Input: dimensioned drawing with shaded views. Units: mm. Origin: part minimum x, y, z. A direction names the side the tool comes from. Round coordinates to 2 decimals unless told otherwise and drop trailing zeros. Loops run counter-clockwise (first coordinate to the right, second up) from the corner with the lowest first, then second, coordinate; pieces in that order, holes last. Notation, with made-up numbers: M 84,16.25 L 138,16.25 A22 cw 138,43.25 Z; hole C 36.5,68.5 d10. An arc over 180 degrees is marked long. One line per item, written item: value.
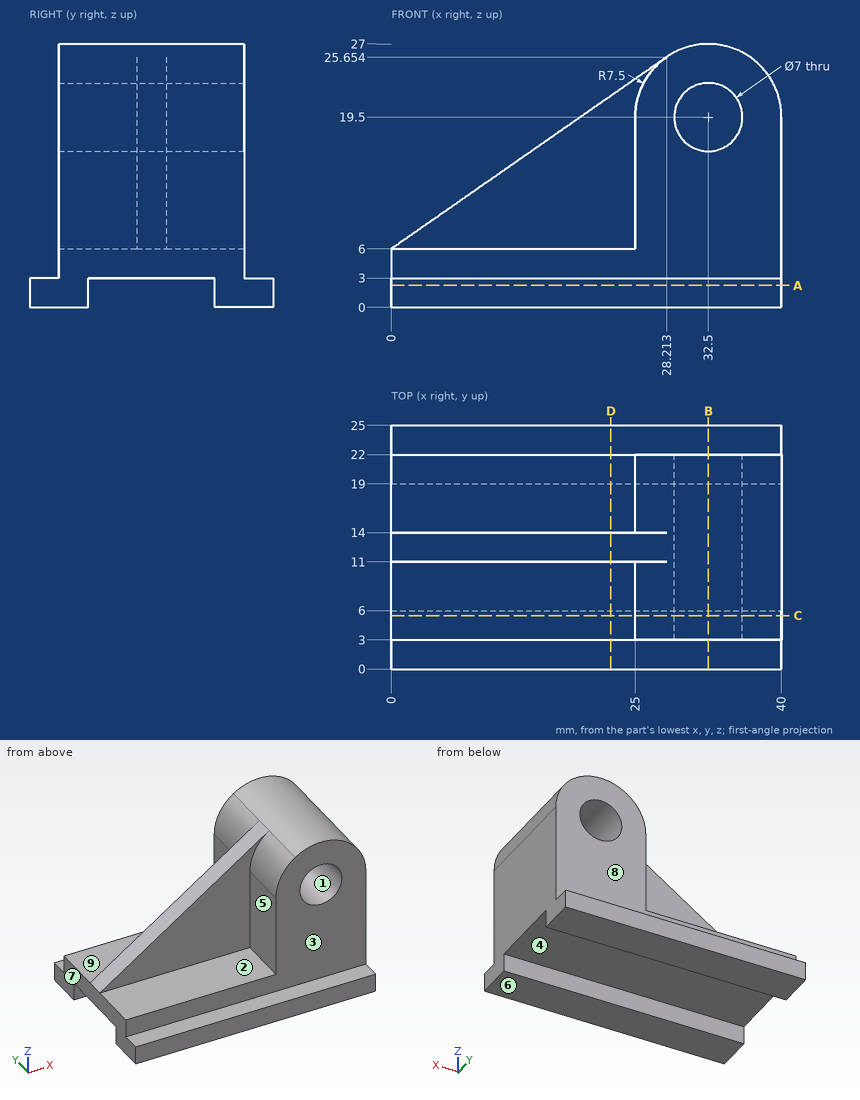
1. Pin query (flat end, axial travel): pin 1 (6.5 mm diameter, centred on y = 5, z = 14.5, fed in from -X); pin 2 (6 mm diameter, centred on x = 16.5, z = 15, fed in from +Y); pin 3 (12 mm diameter, centred on x = 10, z = 20, fed in from -Y); pin 4 (10 mm diameter, centred on y = 4.5, z = 10.5, fed in from -X). Return the tip coordinate at first contact, or that it passes through.
Report:
pin 1: stops at x = 25
pin 2: stops at y = 14
pin 3: stops at y = 11
pin 4: stops at x = 0
2. Section query C-C (y = 5.5). Return the cut outline in (x, z), and give its area (3 significant figures).
Report:
outline: M 0,0 L 40,0 L 40,19.5 A7.5 ccw 28.21,25.65 A7.5 ccw 25,19.5 L 25,6 L 0,6 Z; hole C 32.5,19.5 d7
area: 492 mm2
3. Section query D-D (x = 22.5). Return the cut outline in (y, z), and give its area (3 significant figures).
Report:
outline: M 0,0 L 6,0 L 6,3 L 19,3 L 19,0 L 25,0 L 25,3 L 22,3 L 22,6 L 14,6 L 14,21.67 L 11,21.67 L 11,6 L 3,6 L 3,3 L 0,3 Z
area: 140 mm2
4. Ray query, line 1 (Z direction, x = 32.5, y = 10.75); line 2 (Y direction, x = 12, z = 1); line 3 (Z direction, x = 12.5, y = 1.75). Return the intervals inside material, ascending. Write a range as [from, to].
Report:
line 1: z = [3, 16], [23, 27]
line 2: y = [0, 6], [19, 25]
line 3: z = [0, 3]
5. Section query A-A (z = 2.25). Return the cut outline in (x, y).
Report:
outline: M 0,0 L 40,0 L 40,6 L 0,6 Z; M 0,19 L 40,19 L 40,25 L 0,25 Z
6. Pull-direction query (Z, two-part tool) for the marked faces 1, 2, 3 and 4; classes: released by +Z, released by -Z, zero draft, split by the parting line, or undercut.
Report:
face 1: undercut
face 2: released by +Z
face 3: zero draft
face 4: released by -Z
7. Section query B-B (x = 32.5). Return the cut outline in (y, z).
Report:
outline: M 0,0 L 6,0 L 6,3 L 19,3 L 19,0 L 25,0 L 25,3 L 22,3 L 22,16 L 3,16 L 3,3 L 0,3 Z; M 3,23 L 22,23 L 22,27 L 3,27 Z
8. Reachability of the marked faces 5, 6, 7, 8 and 9 from +Z, -Z, +X, -X, +Y, -Y: full face, straight path, thin tool, end or side. Return the list, or none.
Report:
face 5: +Z, -X, -Y
face 6: -Z, +X, -X, +Y, -Y
face 7: +Z, -Z, -X, +Y, -Y
face 8: +Z, +X, -X, +Y
face 9: +Z, -X, +Y
